Could you check a few things on this model? Use its own coordinates, in mm. Round coordinates to 2 decimals unless told otherwise and drop trailing zeros. One line per question, with ' | ' between items. Start each with the question number.
1. Imagine slicing it at A-A, the plane y = 1.25. State how many separate pieces and enclosed holes the cut face has, and give its area (3 significant figures).
2. For pin 1 Ø3.5 at (x, z) = (276.38, 12.89) entering from -Y, with a flat end and sliding along its axis, tell me the tip position at first contact or that it passes through.
3. If I drill on line 1 along X through (y, z) = (2.2, 73); line 2 along Z through (x, y) = (67, 1.15); line 3 along Z through (x, y) = (158, 1.9), over which ranges is the centre line in solid material (lowest first)? Write a range as [from, to].
from build123d import *

# Parameters (mm, degrees)
ESQUISSE2_W             = 318.15
ESQUISSE2_H             = 148.59
BOSS_EXTRU_1_DEPTH      = 5
ESQUISSE3_R             = 2
ENL_V_MAT_EXTRU_1_DEPTH = 5
ENL_V_MAT_EXTRU_2_DEPTH = 5
ENL_V_MAT_EXTRU_3_DEPTH = 5
ESQUISSE7_W             = 10
ESQUISSE7_H             = 10
ENL_V_MAT_EXTRU_4_DEPTH = 5


with BuildPart() as part:
    # Esquisse2 → Boss.-Extru.1 (new body)
    with BuildSketch(Plane(origin=(0, 0, 0), x_dir=(1, 0, 0), z_dir=(0, 1, 0))):
        with Locations((127.309454852, -77.182817805)):
            Rectangle(ESQUISSE2_W, ESQUISSE2_H)
    extrude(amount=BOSS_EXTRU_1_DEPTH)

    # Esquisse3 → Enlèv. mat.-Extru.1 (cut)
    with BuildSketch(Plane(origin=(0, 5, 0), x_dir=(1, 0, 0), z_dir=(0, 1, 0))):
        with Locations(Location((276.384454852, -141.477817805, 0), (0, 0, 270))):
            Circle(ESQUISSE3_R)
        with Locations(Location((276.384454852, -12.887817805, 0), (0, 0, 270))):
            Circle(ESQUISSE3_R)
        with Locations(Location((-21.765545148, -12.887817805, 0), (0, 0, 270))):
            Circle(ESQUISSE3_R)
        with Locations(Location((-21.765545148, -141.477817805, 0), (0, 0, 270))):
            Circle(ESQUISSE3_R)
    extrude(amount=-ENL_V_MAT_EXTRU_1_DEPTH, mode=Mode.SUBTRACT)

    # Esquisse4 → Enlèv. mat.-Extru.2 (cut)
    with BuildSketch(Plane(origin=(0, 5, 0), x_dir=(1, 0, 0), z_dir=(0, 1, 0))):
        Polygon((73.982481978, -83.682817805), (73.982481978, -77.182817805), (56.982481978, -77.182817805), (49.982481978, -77.182817805), (49.982481978, -83.682817805), align=None)
        Polygon((56.982481978, -77.182817805), (73.982481978, -77.182817805), (73.982481978, -70.682817805), (49.982481978, -70.682817805), (49.982481978, -77.182817805), align=None)
    extrude(amount=-ENL_V_MAT_EXTRU_2_DEPTH, mode=Mode.SUBTRACT)

    # Esquisse6 → Enlèv. mat.-Extru.3 (cut)
    with BuildSketch(Plane(origin=(0, 0, 0), x_dir=(-1, 0, 0), z_dir=(0, -1, 0))):
        with BuildLine():
            Line((-161.982481978, -37.182817805), (-141.982481978, -37.182817805))
            add(Edge.make_bspline(
                [(-141.982481978, -117.182817805), (-181.982481978, -77.182817805), (-141.982481978, -37.182817805)],
                knots=[0, 0, 0, 1, 1, 1], degree=2))
            Line((-141.982481978, -117.182817805), (-161.982481978, -117.182817805))
            add(Edge.make_bspline(
                [(-161.982481978, -117.182817805), (-201.982481978, -77.182817805), (-161.982481978, -37.182817805)],
                knots=[0, 0, 0, 1, 1, 1], degree=2))
        make_face()
    extrude(amount=-ENL_V_MAT_EXTRU_3_DEPTH, mode=Mode.SUBTRACT)

    # Esquisse7 → Enlèv. mat.-Extru.4 (cut)
    with BuildSketch(Plane(origin=(0, 0, 0), x_dir=(-1, 0, 0), z_dir=(0, -1, 0))):
        with Locations((6.765545148, -77.182817805)):
            Rectangle(ESQUISSE7_W, ESQUISSE7_H)
    extrude(amount=-ENL_V_MAT_EXTRU_4_DEPTH, mode=Mode.SUBTRACT)


solid = part.part
Geometry results:
1) separate pieces: 1 | enclosed holes: 7 | area: 45,200 mm2
2) pin 1: passes through
3) line 1: x = [-31.77, -11.77], [-1.77, 49.98], [73.98, 161.76], [181.76, 286.38] | line 2: z = [2.89, 70.68], [83.68, 151.48] | line 3: z = [2.89, 37.18], [59.33, 95.03], [117.18, 151.48]
